Verification items for the finished model (mm, model axes). A direction names the side the tool comes from. Round coordinates to 2 decimals unless told otherwise and drop trailing zeros. Write each loop counter-clockwise with the first axis right and the second up, starting at its lowest first coordinate (ties: lowest second). Pieces come first, ordered by that corner, then holes. Notation, with made-up numbers: M -15.5,-34.75 L 31.5,-34.75 A31 ccw 31.5,-1.75 Z; hole C 27.25,60.5 d11. An arc over 180 degrees is marked long. One line per question, with ' | ' between items. Start each with the question number.
Q1. Cross-section at C-C (z = 7.5). Record the boundary of the cut face in (x, y), then the cut area to 3 significant figures.
Q2. Gauge pin test, flat ends, axial feed: pin 1 (4 mm diameter, centred on y = -4, z = 17.5, fed in from -X); pin 2 (2 mm diameter, centred on x = -12, z = 27, fed in from +Y); pin 3 (1 mm diameter, centred on x = -41, z = 28, fed in from +Y). Record the tip position at first contact, or that the pin passes through.
Q3. Release check for a two-part mould opening along Y. For faces 1 (the face through (25, 1, 30)), 2 (the face through (-10, 0, 15)), 3 (the face through (-59.94, 2.64, 14.82)) record: released by +Y, released by -Y, zero draft, split by the parting line, or undercut.
Q4. Thickness scan on line 1 along Y through (x, z) = (0, 6); line 2 along Z through (x, y) = (39, 33); line 3 along Z through (x, y) = (-20, 0.5). Record the ranges inside material, lowest first. Write a range as from..to.
Q5. Cross-section at A-A (y = 0). Record the boundary of the cut face in (x, z).
Q6. Tool access check on faces 4 (the face through (-5, -9, -3)), 5 (the face through (25, 1, 0)). Record the directions out of +Z, -Z, +X, -X, +Y, -Y that give a thin tool (end or side, any length) a straight path to the whole face; none if there is none.
from build123d import *

# Parameters (mm, degrees)
SKETCH1_R           = 60
BOSS_EXTRUDE1_DEPTH = 30
FILLET1_R           = 2
SKETCH6_R           = 20
BOSS_EXTRUDE6_DEPTH = 3
SKETCH9_R           = 10
CUT_EXTRUDE3_DEPTH  = 92.043945535
FILLET4_R           = 5
SKETCH12_R          = 20
BOSS_EXTRUDE9_DEPTH = 3
FILLET7_R           = 5
SKETCH14_R          = 10
CUT_EXTRUDE5_DEPTH  = 93.17374904


with BuildPart() as part:
    # Sketch1 → Boss-Extrude1 (new body)
    with BuildSketch(Plane.XY):
        Circle(SKETCH1_R)
    extrude(amount=BOSS_EXTRUDE1_DEPTH)

    # Fillet1
    fillet1_edges = [part.edges().sort_by_distance(p)[0] for p in [
        (-60, 0, 0),
        (-60, 0, 30),
    ]]
    fillet(fillet1_edges, radius=FILLET1_R)

    # Sketch6 → Boss-Extrude6 (add)
    with BuildSketch(Plane.XY.offset(30)):
        Circle(SKETCH6_R)
    extrude(amount=BOSS_EXTRUDE6_DEPTH)

    # Sketch9 → Cut-Extrude3 (cut, through all)
    with BuildSketch(Plane.XY.offset(33)):
        Circle(SKETCH9_R)
    extrude(amount=-CUT_EXTRUDE3_DEPTH, mode=Mode.SUBTRACT)

    # Fillet4
    # the kernel refuses this fillet: 5 mm, written as the material it adds along each edge
    with BuildSketch(Plane(origin=(0, 0, 30), x_dir=(1, 0, 0), z_dir=(0, -1, 0))) as fillet4_piece_1:
        with BuildLine():
            CenterArc((24.582575695, 5), FILLET4_R, 203.578178478, 66.421821522)
            Line((20, 3), (19.908348486, 2.96))
            ThreePointArc((19.908348486, 2.96), (19.9, 1.5), (19.9, 0))
            Line((19.9, 0), (20, -0.1))
            Line((20, -0.1), (24.582575695, -0.1))
            Line((24.582575695, -0.1), (24.582575695, 0))
        make_face()
    revolve(axis=Axis((0, 0, 30), (0, 0, 1)))

    # Sketch12 → Boss-Extrude9 (add)
    with BuildSketch(Plane(origin=(0, 0, 0), x_dir=(-1, 0, 0), z_dir=(0, 0, -1))):
        with Locations(Location((0, 0, 0), (0, 0, 180))):
            Circle(SKETCH12_R)
    extrude(amount=BOSS_EXTRUDE9_DEPTH)

    # Fillet7
    # the kernel refuses this fillet: 5 mm, written as the material it adds along each edge
    with BuildSketch(Plane(origin=(0, 0, 0), x_dir=(1, 0, 0), z_dir=(0, 1, 0))) as fillet7_piece_1:
        with BuildLine():
            CenterArc((24.582575695, 5), FILLET7_R, 203.578178478, 66.421821522)
            Line((20, 3), (19.908348486, 2.96))
            ThreePointArc((19.908348486, 2.96), (19.9, 1.5), (19.9, 0))
            Line((19.9, 0), (20, -0.1))
            Line((20, -0.1), (24.582575695, -0.1))
            Line((24.582575695, -0.1), (24.582575695, 0))
        make_face()
    revolve(axis=Axis((0, 0, 0), (0, 0, -1)))

    # Sketch14 → Cut-Extrude5 (cut, through all)
    with BuildSketch(Plane(origin=(0, 0, -3), x_dir=(-1, 0, 0), z_dir=(0, 0, -1))):
        with Locations(Location((0, 0, 0), (0, 0, 180))):
            Circle(SKETCH14_R)
    extrude(amount=-CUT_EXTRUDE5_DEPTH, mode=Mode.SUBTRACT)


solid = part.part
Determined:
1) outline: C 0,0 d120; hole C 0,0 d20 | area: 11,000 mm²
2) pin 1: stops at x = -59.97 | pin 2: stops at y = 58.98 | pin 3: stops at y = 44.27
3) face 1: zero draft | face 2: undercut | face 3: split by the parting line
4) line 1: y = -60..-10, 10..60 | line 2: z = 0..30 | line 3: z = -2.99..32.99
5) outline: M -60,2 A2 ccw -58,0 L -24.58,0 A5 cw -20,-3 L -10,-3 L -10,33 L -20,33 A5 cw -24.58,30 L -58,30 A2 ccw -60,28 Z; M 10,-3 L 20,-3 A5 cw 24.58,0 L 58,0 A2 ccw 60,2 L 60,28 A2 ccw 58,30 L 24.58,30 A5 cw 20,33 L 10,33 Z
6) face 4: -Z, +X, -X, +Y, -Y | face 5: -Z
